Source: CAD feature listing. Evaluate the final solid. Frame: model axes, mm. Coordinates: 2 decimals unless noted, no trailing zeros. Write each loop counter-clockwise with the first axis right and the second up, starting at its lowest first coordinate (ties: lowest second). Pieces come first, ordered by that corner, then holes. Notation, with made-up numbers: (40.25, 1.25) - (98.25, 1.25) arc R26 cw to (98.25, 15.25) - close; hole circle Ø9 at (49.5, 21). An arc over 180 degrees is marked (long way). One line per item, written item: value.
from build123d import *

# Parameters (mm, degrees)
SKETCH1_W           = 139.7
SKETCH1_H           = 127
SKETCH1_R           = 2.5527
BOSS_EXTRUDE1_DEPTH = 2.286
SKETCH2_R           = 1.89865
CUT_EXTRUDE1_DEPTH  = 3.286
FILLET1_R           = 0.635
SKETCH4_R           = 1.89865
CUT_EXTRUDE3_DEPTH  = 3.286


with BuildPart() as part:
    # Sketch1 → Boss-Extrude1 (new body)
    with BuildSketch(Plane(origin=(0, 0, 0), x_dir=(1, 0, 0), z_dir=(0, 1, 0))):
        Rectangle(SKETCH1_W, SKETCH1_H)
        with Locations((-15.875, 25.4)):
            Circle(SKETCH1_R, mode=Mode.SUBTRACT)
        with Locations((3.175, 25.4)):
            Circle(SKETCH1_R, mode=Mode.SUBTRACT)
        with Locations((-15.875, -25.4)):
            Circle(SKETCH1_R, mode=Mode.SUBTRACT)
        with Locations((3.175, -25.4)):
            Circle(SKETCH1_R, mode=Mode.SUBTRACT)
        with Locations((-27.2034, 25.4)):
            Circle(SKETCH1_R, mode=Mode.SUBTRACT)
        with Locations((14.5034, 25.4)):
            Circle(SKETCH1_R, mode=Mode.SUBTRACT)
        with Locations((14.5034, -25.4)):
            Circle(SKETCH1_R, mode=Mode.SUBTRACT)
        with Locations((-27.2034, -25.4)):
            Circle(SKETCH1_R, mode=Mode.SUBTRACT)
        with Locations((52.6034, 25.4)):
            Circle(SKETCH1_R, mode=Mode.SUBTRACT)
        with Locations((52.6034, -25.4)):
            Circle(SKETCH1_R, mode=Mode.SUBTRACT)
    extrude(amount=BOSS_EXTRUDE1_DEPTH)

    # Sketch2 → Cut-Extrude1 (cut, through all)
    with BuildSketch(Plane.XZ):
        with Locations((0, 58.7375)):
            Circle(SKETCH2_R)
        with Locations((-65.0875, 49.2125)):
            Circle(SKETCH2_R)
        with Locations((65.0875, 49.2125)):
            Circle(SKETCH2_R)
        with Locations((-65.0875, 0)):
            Circle(SKETCH2_R)
        with Locations((65.0875, 0)):
            Circle(SKETCH2_R)
        with Locations((52.3875, 58.7375)):
            Circle(SKETCH2_R)
        with Locations((-26.9875, 58.7375)):
            Circle(SKETCH2_R)
        with Locations((-26.9875, -58.7375)):
            Circle(SKETCH2_R)
        with Locations((52.3875, -58.7375)):
            Circle(SKETCH2_R)
        with Locations((65.0875, -49.2125)):
            Circle(SKETCH2_R)
        with Locations((-65.0875, -49.2125)):
            Circle(SKETCH2_R)
        with Locations((0, -58.7375)):
            Circle(SKETCH2_R)
    extrude(amount=-CUT_EXTRUDE1_DEPTH, mode=Mode.SUBTRACT)

    # Fillet1
    fillet1_edges = [part.edges().sort_by_distance(p)[0] for p in [
        (69.85, 1.143, 63.5),
        (-69.85, 1.143, 63.5),
        (-69.85, 1.143, -63.5),
        (69.85, 1.143, -63.5),
    ]]
    fillet(fillet1_edges, radius=FILLET1_R)

    # Sketch4 → Cut-Extrude3 (cut, through all)
    with BuildSketch(Plane.XZ):
        with Locations((55.5625, 36.5125)):
            Circle(SKETCH4_R)
        with Locations((55.5625, 14.2875)):
            Circle(SKETCH4_R)
        with Locations((55.5625, -14.2875)):
            Circle(SKETCH4_R)
        with Locations((55.5625, -36.5125)):
            Circle(SKETCH4_R)
    extrude(amount=-CUT_EXTRUDE3_DEPTH, mode=Mode.SUBTRACT)


solid = part.part
1) Section query C-C on y = 1.15. State how many separate pieces and enclosed holes the cut face has, then the cut area to 3 significant figures.
Values found:
separate pieces: 1
enclosed holes: 26
area: 17,400 mm2
2) Material intervals for line 1 (X direction, y = 1.3, z = -25.5); line 2 (X direction, y = 0.75, z = -25); line 3 (Z direction, x = 64, y = 0.35), sorted ascending.
Values found:
line 1: -69.85 to -29.75, -24.65 to -18.43, -13.32 to 0.62, 5.73 to 11.95, 17.05 to 50.05, 55.15 to 69.85
line 2: -69.85 to -29.72, -24.68 to -18.4, -13.35 to 0.65, 5.7 to 11.98, 17.02 to 50.08, 55.12 to 69.85
line 3: -63.5 to -50.77, -47.66 to -1.56, 1.56 to 47.66, 50.77 to 63.5
3) Draft query along X for faces 1 (the cylindrical face through (55.038, 1.127, -26.167)), 2 (the cylindrical face through (-25.83, 1.13, -27.55)). Return one class per face: released by +X, released by -X, zero draft, split by the parting line, or undercut.
Values found:
face 1: undercut
face 2: undercut
4) Section query A-A on z = 0. Output: boundary loops of the cut face in (x, y), then the cut area to 3 significant figures.
Values found:
outline: (-69.85, 0) - (-66.99, 0) - (-66.99, 2.29) - (-69.85, 2.29) - close; (-63.19, 0) - (63.19, 0) - (63.19, 2.29) - (-63.19, 2.29) - close; (66.99, 0) - (69.85, 0) - (69.85, 2.29) - (66.99, 2.29) - close
area: 302 mm2
5) Section query B-B on z = 25.4. Output: boundary loops of the cut face in (x, y).
Values found:
outline: (-69.85, 0) - (-29.76, 0) - (-29.76, 2.29) - (-69.85, 2.29) - close; (-24.65, 0) - (-18.43, 0) - (-18.43, 2.29) - (-24.65, 2.29) - close; (-13.32, 0) - (0.62, 0) - (0.62, 2.29) - (-13.32, 2.29) - close; (5.73, 0) - (11.95, 0) - (11.95, 2.29) - (5.73, 2.29) - close; (17.06, 0) - (50.05, 0) - (50.05, 2.29) - (17.06, 2.29) - close; (55.16, 0) - (69.85, 0) - (69.85, 2.29) - (55.16, 2.29) - close
